```python
from build123d import *

# Parameters (mm, degrees)
SKETCH4_W           = 20
SKETCH4_H           = 85
BOSS_EXTRUDE6_DEPTH = 5
SKETCH5_W           = 20
SKETCH5_H           = 30
BOSS_EXTRUDE7_DEPTH = 7.5
SKETCH6_R           = 4
CUT_EXTRUDE1_DEPTH  = 20
SKETCH7_W           = 15
SKETCH7_H           = 5
BOSS_EXTRUDE8_DEPTH = 10
FILLET2_START       = 7.5
FILLET2_DEPTH       = 5
FILLET2_2_DEPTH     = 5
SKETCH8_R           = 2
CUT_EXTRUDE2_DEPTH  = 48.565743976
CUT_EXTRUDE4_DEPTH  = 15
CHAMFER4_SIZE       = 5
CHAMFER7_SIZE       = 1
CHAMFER8_SIZE       = 1
SKETCH10_R          = 2
SKETCH10_R_2        = 5
CUT_EXTRUDE5_DEPTH  = 49.605555238
CHAMFER9_SIZE       = 4
CUT_EXTRUDE6_REACH  = 50.606
SKETCH11_R          = 32
CHAMFER10_SIZE      = 2


with BuildPart() as part:
    # Sketch4 → Boss-Extrude6 (new body)
    with BuildSketch(Plane(origin=(0, 0, 0), x_dir=(1, 0, 0), z_dir=(0, 1, 0))):
        Rectangle(SKETCH4_W, SKETCH4_H)
    extrude(amount=BOSS_EXTRUDE6_DEPTH)

    # Sketch5 → Boss-Extrude7 (add)
    with BuildSketch(Plane(origin=(0, 5, 0), x_dir=(1, 0, 0), z_dir=(0, 1, 0))):
        with Locations((0, 27.5)):
            Rectangle(SKETCH5_W, SKETCH5_H)
    extrude(amount=BOSS_EXTRUDE7_DEPTH)

    # Sketch6 → Cut-Extrude1 (cut)
    with BuildSketch(Plane(origin=(0, 0, -42.5), x_dir=(-1, 0, 0), z_dir=(0, 0, -1))):
        with Locations((0, 12.5)):
            Circle(SKETCH6_R)
    extrude(amount=-CUT_EXTRUDE1_DEPTH, mode=Mode.SUBTRACT)

    # Sketch7 → Boss-Extrude8 (add)
    with BuildSketch(Plane.ZY.offset(10)):
        with Locations((-20, 10)):
            Rectangle(SKETCH7_W, SKETCH7_H)
    boss_extrude8 = extrude(amount=BOSS_EXTRUDE8_DEPTH)

    # Mirror1: Boss-Extrude8 across plane
    add(boss_extrude8.mirror(Plane(origin=(0, 0, 0), x_dir=(0, 0, 1), z_dir=(1, 0, 0))))

    # Fillet2: read off the stored shape, not the designer's step
    # Fillet2 outline → Fillet2 (cut)
    with BuildSketch(Plane(origin=(0, 0, 0), x_dir=(1, 0, 0), z_dir=(0, 1, 0)).offset(FILLET2_START)):
        with BuildLine():
            ThreePointArc((15, 27.5), (18.535533906, 26.035533906), (20, 22.5))
            Line((20, 22.5), (20, 27.5))
            Line((20, 27.5), (15, 27.5))
        make_face()
        with BuildLine():
            ThreePointArc((-20, 22.5), (-18.535533906, 26.035533906), (-15, 27.5))
            Line((-15, 27.5), (-20, 27.5))
            Line((-20, 27.5), (-20, 22.5))
        make_face()
    extrude(amount=FILLET2_DEPTH, mode=Mode.SUBTRACT)

    # Fillet2 2 outline → Fillet2 2 (add)
    with BuildSketch(Plane(origin=(0, 0, 0), x_dir=(1, 0, 0), z_dir=(0, 1, 0)).offset(FILLET2_START)):
        with BuildLine():
            Line((10, 27.5), (15, 27.5))
            ThreePointArc((15, 27.5), (11.464466094, 28.964466094), (10, 32.5))
            Line((10, 32.5), (10, 27.5))
        make_face()
        with BuildLine():
            ThreePointArc((-10, 32.5), (-11.464466094, 28.964466094), (-15, 27.5))
            Line((-15, 27.5), (-10, 27.5))
            Line((-10, 27.5), (-10, 32.5))
        make_face()
    extrude(amount=FILLET2_2_DEPTH)

    # Sketch8 → Cut-Extrude2 (cut, through all)
    with BuildSketch(Plane.XZ.offset(-7.5)):
        with Locations(Location((-15, -22.5, 0), (0, 0, 270))):
            Circle(SKETCH8_R)
        with Locations(Location((15, -22.5, 0), (0, 0, 270))):
            Circle(SKETCH8_R)
    extrude(amount=-CUT_EXTRUDE2_DEPTH, mode=Mode.SUBTRACT)

    # Sketch9 → Cut-Extrude4 (cut)
    with BuildSketch(Plane(origin=(0, 0, -42.5), x_dir=(-1, 0, 0), z_dir=(0, 0, -1))):
        with BuildLine():
            Line((-10, 7.5), (-10, 0))
            Line((-10, 0), (10, 0))
            Line((10, 0), (10, 7.5))
            ThreePointArc((10, 7.5), (0, 1.319660113), (-10, 7.5))
        make_face()
    extrude(amount=-CUT_EXTRUDE4_DEPTH, mode=Mode.SUBTRACT)

    # Chamfer4
    # the kernel refuses this chamfer: 5 mm, written as the material it adds along each edge
    with BuildSketch(Plane(origin=(0, 12.5, -27.5), x_dir=(-0.7729223177191435, 0.6345006625462793, 0), z_dir=(0.6345006625462793, 0.7729223177191435, 0))) as chamfer4_piece_1_section:
        Polygon((11.180339887 + CHAMFER4_SIZE, 0), (11.180339887, -CHAMFER4_SIZE), (11.180339887, 0), align=None)
    chamfer4_piece_1 = revolve(axis=Axis((0, 12.5, -27.5), (0, 0, 1)), revolution_arc=258.765918747, mode=Mode.PRIVATE)
    chamfer4_piece_1 = split(chamfer4_piece_1, bisect_by=Plane(origin=(-10, 12.5, -27.5), z_dir=(1, 0, 0)), keep=Keep.TOP, mode=Mode.PRIVATE)
    chamfer4_piece_1 = split(chamfer4_piece_1, bisect_by=Plane(origin=(10, 12.5, -27.5), z_dir=(-1, 0, 0)), keep=Keep.TOP, mode=Mode.PRIVATE)
    chamfer4_piece_1 = split(chamfer4_piece_1, bisect_by=Plane(origin=(0, 0, -27.5), z_dir=(0, 1, 0)), keep=Keep.TOP, mode=Mode.PRIVATE)
    chamfer4_piece_1 = split(chamfer4_piece_1, bisect_by=Plane(origin=(0, 12.5, -27.5), z_dir=(0, -1, 0)), keep=Keep.TOP, mode=Mode.PRIVATE)
    add(chamfer4_piece_1)

    # Chamfer7
    chamfer7_edges = [part.edges().sort_by_distance(p)[0] for p in [
        (0, 8.5, -42.5),
    ]]
    chamfer(chamfer7_edges, length=CHAMFER7_SIZE)

    # Chamfer8
    chamfer8_edges = [part.edges().sort_by_distance(p)[0] for p in [
        (0, 1.319660113, -42.5),
        (-10, 10, -42.5),
        (10, 10, -42.5),
    ]]
    chamfer(chamfer8_edges, length=CHAMFER8_SIZE)

    # Sketch10 → Cut-Extrude5 (cut, through all)
    with BuildSketch(Plane.XZ):
        with Locations(Location((-6.1024, 0.209438339, 0), (0, 0, 270))):
            Circle(SKETCH10_R)
        with Locations(Location((6.143458026, 0.226445131, 0), (0, 0, 270))):
            Circle(SKETCH10_R)
        with Locations(Location((6.143458026, 29.773554869, 0), (0, 0, 270))):
            Circle(SKETCH10_R)
        with Locations(Location((-6.1024, 29.790561661, 0), (0, 0, 270))):
            Circle(SKETCH10_R)
        with Locations(Location((0, 15, 0), (0, 0, 270))):
            Circle(SKETCH10_R_2)
    extrude(amount=-CUT_EXTRUDE5_DEPTH, mode=Mode.SUBTRACT)

    # Chamfer9
    chamfer9_edges = [part.edges().sort_by_distance(p)[0] for p in [
        (10, 2.5, 42.5),
        (-10, 2.5, 42.5),
    ]]
    chamfer(chamfer9_edges, length=CHAMFER9_SIZE)

    # Cut-Extrude6: up to this face of the body (flat: up to its plane)
    cut_extrude6_end = Plane(part.part.faces().sort_by_distance((-9.414765004, 5, 13))[0])
    # Sketch11 → Cut-Extrude6 (cut, up to the picked face)
    with BuildSketch(Plane(origin=(0, 12.5, 0), x_dir=(1, 0, 0), z_dir=(0, 1, 0)), mode=Mode.PRIVATE) as cut_extrude6_sk1:
        with Locations((0, -15)):
            Circle(SKETCH11_R)
    cut_extrude6_tool1 = split(extrude(cut_extrude6_sk1.sketch, amount=-CUT_EXTRUDE6_REACH, mode=Mode.PRIVATE), bisect_by=cut_extrude6_end, keep=Keep.BOTH, mode=Mode.PRIVATE)
    add(cut_extrude6_tool1.solids().sort_by(Axis((0, 12.5, 15), (0, -1, 0)))[0], mode=Mode.SUBTRACT)

    # Chamfer10
    chamfer10_edges = [part.edges().sort_by_distance(p)[0] for p in [
        (-20, 10, -12.5),
        (20, 10, -12.5),
    ]]
    chamfer(chamfer10_edges, length=CHAMFER10_SIZE)


solid = part.part
```
The listing builds one solid part. Answer for the finished solid, in the listing's coordinates (mm). A direction names the side the tool comes from. Give positions to 0.01 mm unless a question says otherwise; leave off trailing zeros. Order: outer loops, then holes, each group sorted by start corner. A loop starts at its lowest first (then second) coordinate and runs counter-clockwise, first axis right, second up.
1) Find section D-D on y = 9.75. Give the number of separate pieces and of enclosed holes in the cut face, then the cut area to 3 significant figures.
Reported:
separate pieces: 1
enclosed holes: 2
area: 653 mm2
2) Find section B-B on x = 0. Write down the section's boundary in (y, z), then the cut area to 3 significant figures.
Reported:
outline: (0, -31.18) - (1.32, -32.5) - (1.32, -41.5) - (2.32, -42.5) - (7.5, -42.5) - (8.5, -41.5) - (8.5, -22.5) - (12.5, -22.5) - (12.5, -17) - (5, -17) - (5, 10) - (0, 10) - close; (0, 20) - (5, 20) - (5, 42.5) - (0, 42.5) - close
area: 471 mm2
3) For faces 4 (the face through (-0.17, 1.32, -37.06)), 5 (the face through (15, 7.5, -20)), 6 (the face through (-10, 10, -37)), 7 (the face through (-10, 3, 3)), determine the directions among +Z, -Z, +X, -X, +Y, -Y from which every point of the face is accessible in a straight line to the end or side of a thin tool.
Reported:
face 4: -Z, -Y
face 5: +Z, -Z, +X, -Y
face 6: -Z, -X, +Y, -Y
face 7: +Z, -Z, -X, -Y
4) Determine the mould class of faces 1 (the face through (-0.18, 1.09, -32.27)), 2 (the face through (-7.88, 2.46, -0.71)), 3 (the face through (0.1, 8.5, -32.1)) for opening direction Z: pulls with the +Z half, pulls with the -Z half, needs draft (parallel to the pull), parting line crosses it, or undercut.
Reported:
face 1: pulls with the -Z half
face 2: undercut
face 3: needs draft
5) Find section C-C on z = -11.5. Write down the section's boundary in (x, y).
Reported:
outline: (-10, 0) - (10, 0) - (10, 5) - (-10, 5) - close
6) Given P1, Ø0.5, axis at x = 17.5, y = 10.5, coming from the +Z side; P2, Ø1.5, axis at x = 0, y = 9, coming from the -Z side; P3, Ø4.5, axis at x = 6.14, z = 0.23, coming from the -Y side; P4, Ø2.5, axis at y = 9, z = -38, coming from the +X side, each flat-ended and moving along its own axis, determine where each tip first touches the part or whether it passes through.
Reported:
P1: stops at z = -12.5
P2: stops at z = -41.75
P3: stops at y = 0
P4: stops at x = 10
7) Find section A-A on z = 15. Write down the section's boundary in (x, y), then the cut area to 3 significant figures.
Reported:
outline: (-10, 0) - (-5, 0) - (-5, 5) - (-10, 5) - close; (5, 0) - (10, 0) - (10, 5) - (5, 5) - close
area: 50.0 mm2
8) Consider line 1 along X through (y, z) = (4, 12); line 2 along X through (y, z) = (1.45, 15); line 3 along X through (y, z) = (5.75, -26). Determine where each line is inside the solid, lowest interval first.
Reported:
line 1: x = -10 to -4, 4 to 10
line 2: x = -10 to -5, 5 to 10
line 3: x = -10 to 10
